Autodesk Fusion 360 part; units mm, degrees
sketch "Sketch1" plane through (0, 0, 0) normal (0, 1, 0) x (1, 0, 0)
  line L0 (0, 0) -> (35, -80)
  line L1 (35, -80) -> (65, -80)
  line L2 (65, -80) -> (100, 0)
  line L3 (100, 0) -> (0, 0)
  circle A0 centre (50, -50) radius 7.5
  circle A1 centre (50, -50) radius 3.5
  dimension "d1" = 100
  dimension "d2" = 30
  dimension "d4" = 80
  dimension "d5" = 35
  dimension "d6" = 50
  dimension "d7" = 15
  dimension "d8" = 15
  dimension "d13" = 7
extrude "Extrude1" add sketch "Sketch1" against normal blind 5 contours L0 L1 L2 L3 | A0 | A1
extrude "Extrude2" add sketch "Sketch1" along normal blind 34 contours A0
fillet "Fillet1" radius 9 2 edges at (65, -2.5, 80) (35, -2.5, 80)
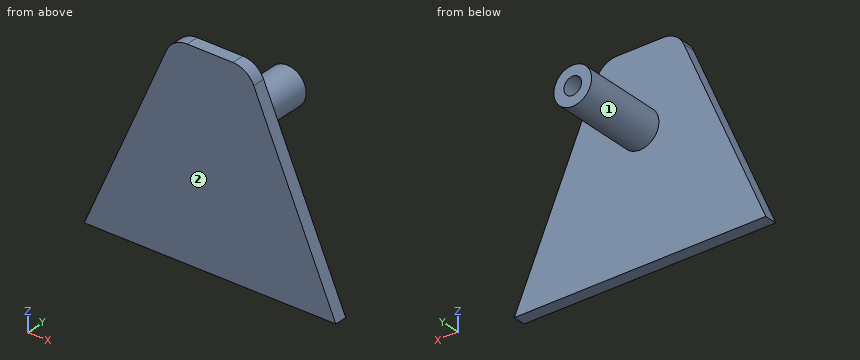
Geometry: final body of the model. Coordinates: model frame, mm. Face numbers are marked on the shaded views. A direction names the side the tool comes from. Give positions to 0.01 mm unless a question says otherwise; leave off trailing zeros. Order: outer loops, then holes, each group sorted by start corner. A loop starts at its lowest first (then second) coordinate and runs counter-clockwise, first axis right, second up. Notation, with made-up numbers: (6.25, -37) -> (50.25, -37) arc R14 ccw to (50.25, -15) -> close; hole circle Ø11 at (46, 64.25). An arc over 180 degrees is marked (long way). Answer as a JSON object with one key per item and string values.
Q1. First-contact query: pin 1 (10 mm diameter, centred on y = 4, z = 58.5, fed in from -X); pin 2 (10 mm diameter, centred on x = 76, z = 64, fed in from +Y); pin 3 (12 mm diameter, centred on y = 12, z = 31.5, fed in from +X); pin 4 (5 mm diameter, centred on x = 59, y = 27.5, fed in from +Z). Flat tips, straight axial feed; report the tip coordinate or a pass-through.
Entries:
{"pin 1": "stops at x = 24.28", "pin 2": "stops at y = 0", "pin 3": "passes through", "pin 4": "stops at z = 53.74"}
Q2. Section A-A (x = 56). Output: boundary loops of the cut face in (y, z).
Entries:
{"outline": "(-5, 0) -> (0, 0) -> (0, 45.5) -> (34, 45.5) -> (34, 54.5) -> (0, 54.5) -> (0, 80) -> (-5, 80) -> close"}
Q3. Material intervals for probe 1 along X at (y, z) = (15, 50); probe 2 along Y at (x, z) = (36.5, 53.5), sorted ascending.
Entries:
{"probe 1": "x = 42.5 to 46.5, 53.5 to 57.5", "probe 2": "y = -5 to 0"}
Q4. Access query for the marked faces 1 and 2. Directions: +Z, -Z, +X, -X, +Y, -Y. A direction counts if a zero-diameter tool reaches every point of the face in a straight line with its end or side. Return the directions, or none.
Entries:
{"face 1": "+Y", "face 2": "+Z, -Z, +X, -X, -Y"}
Q5. Section C-C (y = 26.5). Output: boundary loops of the cut face in (x, z), plus the area to 3 significant figures.
Entries:
{"outline": "circle Ø15 at (50, 50); hole circle Ø7 at (50, 50)", "area": "138 mm^2"}
Q6. Section B-B (z = 50). Output: boundary loops of the cut face in (x, y) (3 decimals).
Entries:
{"outline": "(21.875, -5) -> (78.125, -5) -> (78.125, 0) -> (57.5, 0) -> (57.5, 34) -> (53.5, 34) -> (53.5, 0) -> (46.5, 0) -> (46.5, 34) -> (42.5, 34) -> (42.5, 0) -> (21.875, 0) -> close"}
Q7. Section D-D (z = 71). Output: boundary loops of the cut face in (x, y).
Entries:
{"outline": "(31.06, -5) -> (68.94, -5) -> (68.94, 0) -> (31.06, 0) -> close"}
